from build123d import *

# Parameters (mm, degrees)
F0_W          = 47.4397577345
F0_H          = 56.4533136785
F1_DEPTH      = 40
F3_DEPTH      = 33
F3_DEPTH_BACK = 33.1
F5_DEPTH      = 33.3
F6_W          = 39.4397577345
F6_H          = 31.9497205708
F7_DEPTH      = 26.6
F7_DEPTH_BACK = 25.8


with BuildPart() as f1:
    # F0 (on Top) → F1 (new body)
    with BuildSketch(Plane.XY):
        Rectangle(F0_W, F0_H)
    extrude(amount=F1_DEPTH)

    # F2 (on Front) → F3 (join, two sides)
    with BuildSketch(Plane.XZ) as f3_sk:
        Polygon((33.3382274703, 34.9497205708), (0, 61.778764094), (-31.1693440729, 34.9497205708), (-28.1035822263, 34.9497205708), (29.8146836554, 34.9497205708), align=None)
    extrude(amount=F3_DEPTH)
    extrude(f3_sk.sketch, amount=-F3_DEPTH_BACK)

    # F4 (on Front) → F5 (cut)
    with BuildSketch(Plane.XZ):
        with BuildLine():
            Line((10.4915505733, 0), (9.8356730979, 15))
            ThreePointArc((9.8356730979, 15), (-0.1643269021, 25), (-10.1643269021, 15))
            Line((-10.1643269021, 15), (-10.1643269021, 0))
            Line((-10.1643269021, 0), (10.4915505733, 0))
        make_face()
    extrude(amount=F5_DEPTH, mode=Mode.SUBTRACT)

    # F6 (on Front) → F7 (cut, two sides)
    with BuildSketch(Plane.XZ) as f7_sk:
        with Locations((0, 15.9748602854)):
            Rectangle(F6_W, F6_H)
    extrude(amount=F7_DEPTH, mode=Mode.SUBTRACT)
    extrude(f7_sk.sketch, amount=-F7_DEPTH_BACK, mode=Mode.SUBTRACT)


solid = f1.part
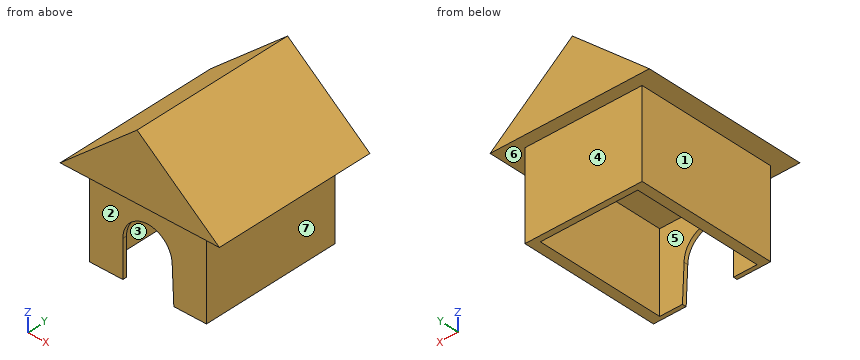
Read the model definition and answer for the solid it produces. Units are mm, in the model's axes. Face numbers are marked on the shaded views. A direction names the side the tool comes from. Round coordinates to 2 decimals unless told otherwise and drop trailing zeros. Order: outer loops, then holes, each group sorted by start corner. A loop starts at its lowest first (then second) coordinate and runs counter-clockwise, first axis right, second up.
1) For the marked faces 1, 2, 3 and 4, determine the directions among +Z, -Z, +X, -X, +Y, -Y from which every point of the face is accessible in a straight line to the end or side of a thin tool.
2) Flat-ended cylindrical pins translate along their axes: pin 1 (0.8 mm diameter, centred on y = -27.5, z = 6.5, fed in from +X); pin 2 (12 mm diameter, centred on x = 26, y = -18, fed in from +Z); pin 3 (9.5 mm diameter, centred on x = -1.5, z = 10, fed in from +Y). Find the tip coordinate at first contact, or state that the pin passes through.
3) The part is cut by section B-B on x = 21.5. Write down the section's boundary in (y, z).
4) The part is cut by section C-C on z = 50. Write down the section's boundary in (x, y), plus the area to 3 significant figures.
5) The part is cut by section D-D on x = -7. Write down the section's boundary in (y, z).
6) The mould has two halves that part along X. Classify the marked faces 5, 6 and 7: released by +X, released by -X, zero draft, split by the parting line, or undercut.
7) Straight lines are drawn through the part: L1, parallel to X at y = -13.5, z = 27; L2, parallel to Y at x = -14, z = 27.5; L3, parallel to X at y = 14.5, z = 33. For each, find the intervals that lie inside material, in ascending order.
8) The part is cut by section A-A on y = 21.5. Write down the section's boundary in (x, z).
Resolved:
1. face 1: -Z, -X, +Y, -Y
1. face 2: -Z, +X, -X, -Y
1. face 3: -Z
1. face 4: -Z, +X, -X, +Y
2. pin 1: stops at x = 23.72
2. pin 2: stops at z = 45.68
2. pin 3: stops at y = 28.23
3. outline: (-33, 34.95) - (-28.23, 34.95) - (-28.23, 0) - (28.23, 0) - (28.23, 34.95) - (33.1, 34.95) - (33.1, 44.48) - (-33, 44.48) - close
4. outline: (-13.68, -33) - (14.64, -33) - (14.64, 33.1) - (-13.68, 33.1) - close
4. area: 1,870 mm2
5. outline: (-33, 34.95) - (-28.23, 34.95) - (-28.23, 22.3) - (-26.6, 22.3) - (-26.6, 31.95) - (25.8, 31.95) - (25.8, 0) - (28.23, 0) - (28.23, 34.95) - (33.1, 34.95) - (33.1, 55.75) - (-33, 55.75) - close
6. face 5: undercut
6. face 6: zero draft
6. face 7: released by +X
7. L1: x = -23.72 to -19.72, 19.72 to 23.72
7. L2: y = -28.23 to -26.6, 25.8 to 28.23
7. L3: x = -23.72 to 23.72
8. outline: (-31.17, 34.95) - (-23.72, 34.95) - (-23.72, 0) - (-19.72, 0) - (-19.72, 31.95) - (19.72, 31.95) - (19.72, 0) - (23.72, 0) - (23.72, 34.95) - (33.34, 34.95) - (0, 61.78) - close
